Geometry: see drawing. Coordinates: mm, zero at the bounding-box minimum. A direction names the side the tool comes from. Round coordinates to 2 decimals unless told otherwise and drop trailing zeros. Loops run counter-clockwise (first coordinate to the right, second up) from the corner with the lowest first, then second, coordinate; pieces in that order, holes last. Notation, with made-up numbers: (49.25, 16.25) - (81.25, 16.25) arc R15 ccw to (81.25, 42.25) - close; hole circle Ø10 at (21, 1). An arc over 180 degrees is marked (long way). Return JSON: item names as keys, results as strings. Group by question number.
1. First-contact query: pin 1 Ø11.5 at (x, y) = (71, 2.5) entering from +Z. Flat tip, straight axial feed; report the tip coordinate or a pass-through.
2. Section B-B on x = 92.5. Return loops of the section in (y, z) (1 decimal).
3. Material intervals for probe 1 along Y at (x, z) = (40, 37.5) (1 decimal); probe 2 along X at (y, z) = (35.5, 31.5) (1 decimal); probe 3 along Y at (x, z) = (129, 31), sorted ascending.
4. Section D-D on y = 49.5. Return loops of the section in (x, z) (1 decimal).
5. Draft query along X for the marked faces 1, 2 and 3. Return one class per face: +X half, -X half, draft (parallel to the pull), parting line (faces both ways), or undercut.
6. Section C-C on z = 47. Return loops of the section in (x, y) (1 decimal), and give its area (3 significant figures).
7. Set-up query: the marked faces 4 and 5. Return all of +Z, -Z, +X, -X, +Y, -Y with unobstructed straight access to the full face (end or side cutting, diameter ignored); none if empty.
8. Section A-A on y = 79. Return loops of the section in (x, z) (1 decimal).
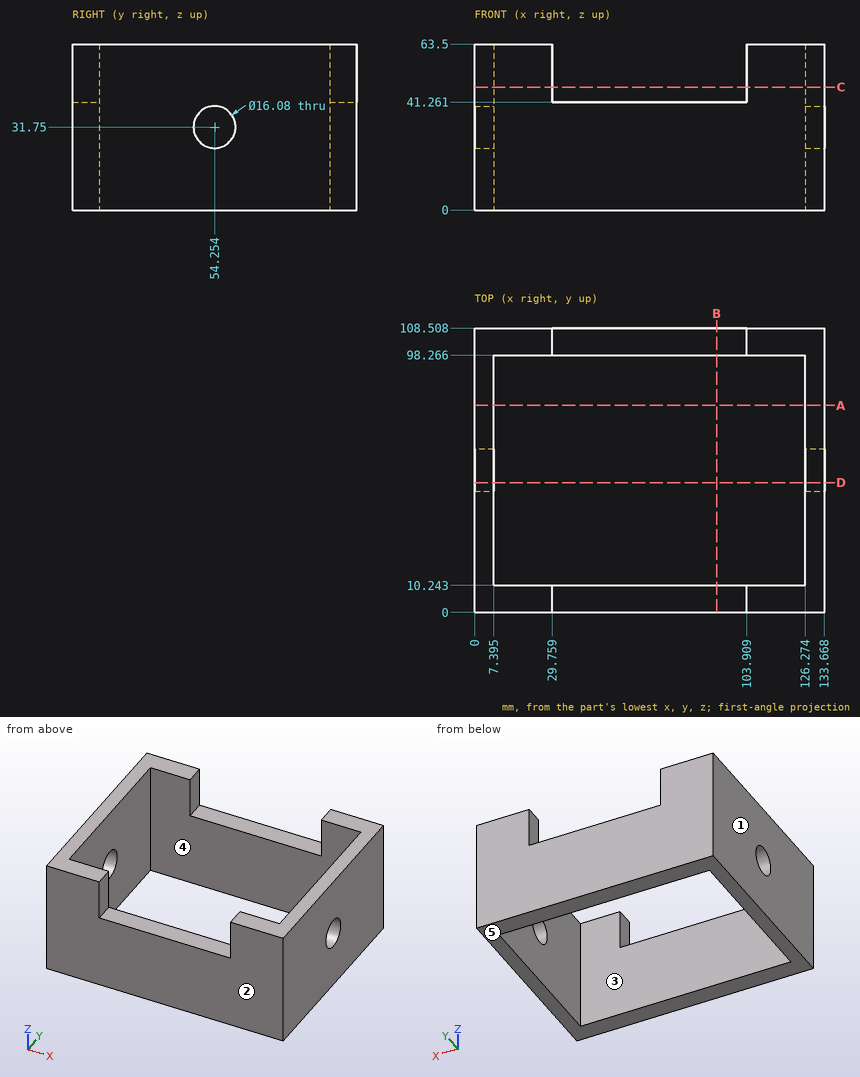
Taken from the geometry:
{
 "1": {"pin 1": "z = 41.26"},
 "2": {"outline": "(0, 0) - (10.2, 0) - (10.2, 41.3) - (0, 41.3) - close; (98.3, 0) - (108.5, 0) - (108.5, 41.3) - (98.3, 41.3) - close"},
 "3": {"probe 1": "0 to 10.2, 98.3 to 108.5", "probe 2": "0 to 7.4, 126.3 to 133.7", "probe 3": "0 to 46.25, 62.26 to 108.51"},
 "4": {"outline": "(0, 0) - (7.4, 0) - (7.4, 25.3) - (0, 25.3) - close; (0, 38.2) - (7.4, 38.2) - (7.4, 63.5) - (0, 63.5) - close; (126.3, 0) - (133.7, 0) - (133.7, 25.3) - (126.3, 25.3) - close; (126.3, 38.2) - (133.7, 38.2) - (133.7, 63.5) - (126.3, 63.5) - close"},
 "5": {"face 1": "-X half", "face 2": "draft", "face 3": "undercut"},
 "6": {"outline": "(0, 0) - (29.8, 0) - (29.8, 10.2) - (7.4, 10.2) - (7.4, 98.3) - (29.8, 98.3) - (29.8, 108.5) - (0, 108.5) - close; (103.9, 0) - (133.7, 0) - (133.7, 108.5) - (103.9, 108.5) - (103.9, 98.3) - (126.3, 98.3) - (126.3, 10.2) - (103.9, 10.2) - close", "area": "2,520 mm2"},
 "7": {"face 4": "+Z, -Z", "face 5": "-Z, +X, -X, +Y, -Y"},
 "8": {"outline": "(0, 0) - (7.4, 0) - (7.4, 63.5) - (0, 63.5) - close; (126.3, 0) - (133.7, 0) - (133.7, 63.5) - (126.3, 63.5) - close"}
}
